Verification items for the finished model (mm, model axes). Coordinates: 2 decimals unless noted, no trailing zeros. Order: outer loops, then holes, each group sorted by start corner. A loop starts at its lowest first (then second) coordinate and runs counter-clockwise, first axis right, second up. Notation, with made-up numbers: M 60,51.5 L 66,51.5 A20 cw 66,84.5 Z; hole C 16,76.25 d2. An arc over 180 degrees is marked long. Use one line per item in the form item = value. Start each with the question number.
```python
from build123d import *

# Parameters (mm, degrees)
SKETCH1_W           = 35.5
SKETCH1_H           = 17.7
SKETCH1_R           = 0.35
BOSS_EXTRUDE1_DEPTH = 1.4


with BuildPart() as part:
    # Sketch1 → Boss-Extrude1 (new body)
    with BuildSketch(Plane(origin=(0, 0, 0), x_dir=(1, 0, 0), z_dir=(0, 1, 0))):
        Rectangle(SKETCH1_W, SKETCH1_H)
        with Locations((-16.51, 7.61)):
            Circle(SKETCH1_R, mode=Mode.SUBTRACT)
        with Locations((-13.97, 7.61)):
            Circle(SKETCH1_R, mode=Mode.SUBTRACT)
        with Locations((-11.43, 7.61)):
            Circle(SKETCH1_R, mode=Mode.SUBTRACT)
        with Locations((-8.89, 7.61)):
            Circle(SKETCH1_R, mode=Mode.SUBTRACT)
        with Locations((-6.35, 7.61)):
            Circle(SKETCH1_R, mode=Mode.SUBTRACT)
        with Locations((-3.81, 7.61)):
            Circle(SKETCH1_R, mode=Mode.SUBTRACT)
        with Locations((-1.27, 7.61)):
            Circle(SKETCH1_R, mode=Mode.SUBTRACT)
        with Locations((1.27, 7.61)):
            Circle(SKETCH1_R, mode=Mode.SUBTRACT)
        with Locations((3.81, 7.61)):
            Circle(SKETCH1_R, mode=Mode.SUBTRACT)
        with Locations((6.35, 7.61)):
            Circle(SKETCH1_R, mode=Mode.SUBTRACT)
        with Locations((8.89, 7.61)):
            Circle(SKETCH1_R, mode=Mode.SUBTRACT)
        with Locations((11.43, 7.61)):
            Circle(SKETCH1_R, mode=Mode.SUBTRACT)
        with Locations((13.97, 7.61)):
            Circle(SKETCH1_R, mode=Mode.SUBTRACT)
        with Locations((16.51, 7.61)):
            Circle(SKETCH1_R, mode=Mode.SUBTRACT)
        with Locations((16.51, -7.61)):
            Circle(SKETCH1_R, mode=Mode.SUBTRACT)
        with Locations((13.97, -7.61)):
            Circle(SKETCH1_R, mode=Mode.SUBTRACT)
        with Locations((11.43, -7.61)):
            Circle(SKETCH1_R, mode=Mode.SUBTRACT)
        with Locations((8.89, -7.61)):
            Circle(SKETCH1_R, mode=Mode.SUBTRACT)
        with Locations((6.35, -7.61)):
            Circle(SKETCH1_R, mode=Mode.SUBTRACT)
        with Locations((3.81, -7.61)):
            Circle(SKETCH1_R, mode=Mode.SUBTRACT)
        with Locations((1.27, -7.61)):
            Circle(SKETCH1_R, mode=Mode.SUBTRACT)
        with Locations((-1.27, -7.61)):
            Circle(SKETCH1_R, mode=Mode.SUBTRACT)
        with Locations((-3.81, -7.61)):
            Circle(SKETCH1_R, mode=Mode.SUBTRACT)
        with Locations((-6.35, -7.61)):
            Circle(SKETCH1_R, mode=Mode.SUBTRACT)
        with Locations((-8.89, -7.61)):
            Circle(SKETCH1_R, mode=Mode.SUBTRACT)
        with Locations((-11.43, -7.61)):
            Circle(SKETCH1_R, mode=Mode.SUBTRACT)
        with Locations((-13.97, -7.61)):
            Circle(SKETCH1_R, mode=Mode.SUBTRACT)
        with Locations((-16.51, -7.61)):
            Circle(SKETCH1_R, mode=Mode.SUBTRACT)
        with Locations((-13.97, 5.07)):
            Circle(SKETCH1_R, mode=Mode.SUBTRACT)
        with Locations((16.51, 5.07)):
            Circle(SKETCH1_R, mode=Mode.SUBTRACT)
        with Locations((16.51, 2.53)):
            Circle(SKETCH1_R, mode=Mode.SUBTRACT)
        with Locations((16.51, -0.01)):
            Circle(SKETCH1_R, mode=Mode.SUBTRACT)
        with Locations((16.51, -2.55)):
            Circle(SKETCH1_R, mode=Mode.SUBTRACT)
        with Locations((16.51, -5.09)):
            Circle(SKETCH1_R, mode=Mode.SUBTRACT)
    extrude(amount=BOSS_EXTRUDE1_DEPTH)


solid = part.part
```
1. Material ranges on line 1 along Z through (x, y) = (-3.81, 0.35); line 2 along X through (y, z) = (0.9, -5.07); line 3 along Z through (x, y) = (-14, 0.45), recorded low to high.
2. Cross-section at A-A on x = 16.51. Give the number of separate pieces and of enclosed holes in the cut face, and give its area (3 significant figures).
3. Cross-section at D-D on z = 2.55. Enter the section's corners in (x, y).
4. Cross-section at B-B on z = -5.07. Enter the section's corners in (x, y), and give its area (3 significant figures).
5. Cross-section at C-C on x = -13.97. Enter the section's corners in (y, z), and give its area (3 significant figures).
Final values:
q1.line_1 = -8.85 to -7.96, -7.26 to 7.26, 7.96 to 8.85
q1.line_2 = -17.75 to -14.32, -13.62 to 16.16, 16.86 to 17.75
q1.line_3 = -8.85 to -7.96, -7.26 to -5.42, -4.72 to 7.26, 7.96 to 8.85
q2.separate_pieces = 8
q2.enclosed_holes = 0
q2.area = 17.9 mm2
q3.outline = M -17.75,0 L 16.16,0 L 16.16,1.4 L -17.75,1.4 Z; M 16.86,0 L 17.75,0 L 17.75,1.4 L 16.86,1.4 Z
q4.outline = M -17.75,0 L -14.32,0 L -14.32,1.4 L -17.75,1.4 Z; M -13.62,0 L 16.16,0 L 16.16,1.4 L -13.62,1.4 Z; M 16.86,0 L 17.75,0 L 17.75,1.4 L 16.86,1.4 Z
q4.area = 47.7 mm2
q5.outline = M 0,-8.85 L 1.4,-8.85 L 1.4,-7.96 L 0,-7.96 Z; M 0,-7.26 L 1.4,-7.26 L 1.4,-5.42 L 0,-5.42 Z; M 0,-4.72 L 1.4,-4.72 L 1.4,7.26 L 0,7.26 Z; M 0,7.96 L 1.4,7.96 L 1.4,8.85 L 0,8.85 Z
q5.area = 21.8 mm2
